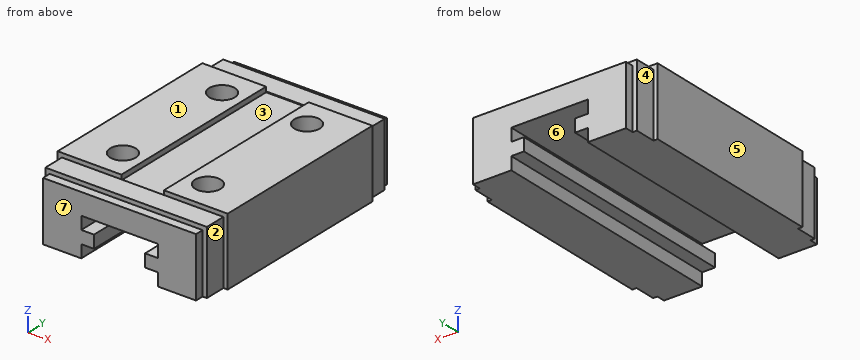
Autodesk Inventor part; units mm, degrees
ref_plane "YZ Plane" through (0, 0, 0) normal (1, 0, 0) x (0, 1, 0)
ref_plane "XZ Plane" through (0, 0, 0) normal (0, 1, 0) x (-1, 0, 0)
ref_plane "XY Plane" through (0, 0, 0) normal (0, 0, 1) x (1, 0, 0)
sketch "Szkic1" plane through (0, 0, 0) normal (0, 0, 1) x (1, 0, 0)
  line L0 (0, 0) -> (10, 0)
  line L1 (10, 0) -> (10, 28.9)
  line L2 (10, 28.9) -> (-10, 28.9)
  line L3 (-10, 28.9) -> (-10, 0)
  line L4 (-10, 0) -> (10, 0)
  dimension "d1" = 28.9
  dimension "d2" = 20
extrude "Wyciągnięcie proste1" add sketch "Szkic1" along normal blind 8
sketch "Szkic2" plane through (-10, 0, 0) normal (0, -1, 0) x (1, 0, 0)
  line L0 (0, 0) -> (20, 0)
  line L1 (20, 0) -> (20, 8)
  line L2 (0, 8) -> (20, 8)
  line L3 (0, 0) -> (0, 8)
  line L4 (14.5, 4.5) -> (5.5, 4.5)
  line L5 (14.5, 4.5) -> (14.5, 3)
  line L6 (14.5, 3) -> (13, 3)
  line L7 (13, 3) -> (13, 1.5)
  line L8 (13, 1.5) -> (14.5, 1.5)
  line L9 (5.5, 4.5) -> (5.5, 3)
  line L10 (5.5, 3) -> (7, 3)
  line L11 (7, 3) -> (7, 1.5)
  line L12 (7, 1.5) -> (5.5, 1.5)
  line L13 (5.5, 4.5) -> (5.5, 3)
  line L14 (5.5, 1.5) -> (5.5, 0)
  line L15 (14.5, 0) -> (14.5, 1.5)
  line L16 (14.5, 3) -> (14.5, 4.5)
extrude "Wyciągnięcie proste2" cut sketch "Szkic2" against normal up to next contours L14 L12 L11 L10 L9 L4 L5 L6 L7 L8 L15 L0
sketch "Szkic3" plane through (0, 0, 8) normal (0, 0, 1) x (1, 0, 0)
  line L0 (10, 0) -> (10, 28.9)
  line L1 (10, 28.9) -> (-10, 28.9)
  line L2 (-10, 28.9) -> (-10, 0)
  line L3 (-10, 0) -> (10, 0)
  line L4 (10, 28.9) -> (-10, 0)
  line L5 (10, 28.9) -> (-10, 28.9)
  line L6 (10, 0) -> (-10, 28.9)
  line L7 (-10, 28.9) -> (0, 14.45)
  line L8 (0, 14.45) -> (0, 6.95)
  line L9 (0, 6.95) -> (5, 6.95)
  line L10 (5, 6.95) -> (5, 21.95)
  line L11 (3, 0) -> (3, 28.9)
  line L12 (5, 21.95) -> (-5, 21.95)
  line L13 (-5, 21.95) -> (-5, 6.95)
  line L14 (-5, 6.95) -> (0, 6.95)
  line L15 (-3, 0) -> (-3, 28.9)
  circle A0 centre (5, 21.95) radius 1.5
  circle A1 centre (5, 6.95) radius 1.5
  circle A2 centre (-5, 21.95) radius 1.5
  circle A3 centre (-5, 6.95) radius 1.5
  point P0 (0, 0)
  dimension "d23" = 10
  dimension "d24" = 15
  dimension "d25" = 3
  dimension "d26" = 3
  dimension "d27" = 3
  dimension "d28" = 3
extrude "Wyciągnięcie proste3" cut sketch "Szkic3" against normal blind 3 contours A1 L9 L10 L6 | L6 L10 A1 | A0 L10 L4 | L4 L10 L12 A0 | L10 L9 A1 L6 | L6 A1 L10 | L10 A0 L4 | L4 A0 L12 L10 | A3 L13 L4 | L4 L13 L14 A3 | L14 L13 L4 A3 | A2 L12 L13 L6 | L6 L13 A2 | A2 L6 L13 L12 | L13 A3 L4 | L6 A2 L13
thread "Gwint1"
thread "Gwint2"
thread "Gwint3"
thread "Gwint4"
sketch "Szkic4" plane through (0, 0, 8) normal (0, 0, 1) x (1, 0, 0)
  circle A0 centre (-5, 6.95) radius 1.5
  circle A1 centre (5, 6.95) radius 1.5
  circle A2 centre (5, 21.95) radius 1.5
  circle A3 centre (-5, 21.95) radius 1.5
  line L0 (10, 28.9) -> (-10, 28.9)
  line L1 (-10, 0) -> (10, 0)
  line L2 (-10, 0) -> (-10, 1)
  line L3 (-10, 1) -> (10, 1)
  line L4 (-10, 28.9) -> (-10, 27.9)
  line L5 (-10, 27.9) -> (10, 27.9)
  line L6 (-10, 28.9) -> (-10, 27.9)
  line L7 (-10, 1) -> (-10, 0)
  line L8 (10, 0) -> (10, 1)
  line L9 (10, 27.9) -> (10, 28.9)
  line L10 (10, 0) -> (10, 1)
  line L11 (10, 27.9) -> (10, 28.9)
  line L12 (-10, 28.9) -> (-10, 27.9)
  line L13 (-10, 1) -> (-10, 0)
  point P0 (0, 0)
  dimension "d39" = 1
  dimension "d40" = 1
extrude "Wyciągnięcie proste4" cut sketch "Szkic4" against normal blind 1 contours L9 L5 L4 L0 | L2 L3 L8 L1
sketch "Szkic5" plane through (10, 0, 0) normal (1, 0, 0) x (0, 0, -1)
  line L0 (-7, 1) -> (-7, 0)
  line L1 (0, 0) -> (-7, 0)
  line L2 (0, 0) -> (0, 28.9)
  line L3 (-7, 28.9) -> (-7, 27.9)
  line L4 (0, 28.9) -> (-7, 28.9)
  line L5 (-7, 1) -> (0, 1)
  line L6 (-7, 27.9) -> (0, 27.9)
extrude "Wyciągnięcie proste5" cut sketch "Szkic5" against normal blind 1
sketch "Szkic6" plane through (-10, 0, 0) normal (-1, 0, 0) x (0, 0, 1)
  line L0 (7, 27.9) -> (7, 28.9)
  line L1 (0, 28.9) -> (7, 28.9)
  line L2 (0, 28.9) -> (0, 0)
  line L3 (0, 0) -> (7, 0)
  line L4 (7, 0) -> (7, 1)
  line L5 (8, 27.9) -> (7, 27.9)
  line L6 (7, 27.9) -> (0, 27.9)
  line L7 (7, 1) -> (0, 1)
extrude "Wyciągnięcie proste6" cut sketch "Szkic6" against normal blind 1
sketch "Szkic7" plane through (0, 0, 8) normal (0, 0, 1) x (1, 0, 0)
  circle A0 centre (-5, 21.95) radius 1.5
  circle A1 centre (5, 21.95) radius 1.5
  circle A2 centre (5, 6.95) radius 1.5
  circle A3 centre (-5, 6.95) radius 1.5
  line L0 (-10, 1) -> (10, 1)
  line L1 (10, 27.9) -> (-10, 27.9)
  line L2 (10, 27.9) -> (10, 25.4)
  line L3 (10, 25.4) -> (-10, 25.4)
  line L4 (10, 1) -> (9, 1)
  line L5 (10, 1) -> (10, 3.5)
  line L6 (10, 3.5) -> (-10, 3.5)
  line L7 (10, 1) -> (10, 3.5)
  line L8 (10, 25.4) -> (10, 27.9)
  line L9 (10, 1) -> (10, 3.5)
  line L10 (10, 25.4) -> (10, 27.9)
  line L11 (-10, 27.9) -> (-10, 25.4)
  line L12 (-10, 3.5) -> (-10, 1)
  line L13 (-10, 27.9) -> (-10, 25.4)
  line L14 (-10, 3.5) -> (-10, 1)
  point P0 (0, 0)
  dimension "d47" = 2.5
  dimension "d48" = 2.5
extrude "Wyciągnięcie proste7" cut sketch "Szkic7" against normal blind 0.5 contours L12 L6 L5 L0 | L2 L3 L11 L1
sketch "Szkic8" plane through (-10, 1, 0) normal (-1, 0, 0) x (0, 0, 1)
  line L0 (7.5, 24.4) -> (7.5, 26.9)
  line L1 (7.5, 26.9) -> (0, 26.9)
  line L2 (7.5, 0) -> (7.5, 2.5)
  line L3 (0, 0) -> (7.5, 0)
  line L4 (0, 26.9) -> (0, 0)
  line L5 (7.5, 24.4) -> (0, 24.4)
  line L6 (7.5, 2.5) -> (7.5, 0)
  line L7 (7.5, 2.5) -> (0, 2.5)
  point P0 (0, -1)
extrude "Wyciągnięcie proste8" cut sketch "Szkic8" against normal blind 0.5
sketch "Szkic9" plane through (10, 1, 0) normal (1, 0, 0) x (0, 0, -1)
  line L0 (-7.5, 2.5) -> (-7.5, 0)
  line L1 (-7.5, 0) -> (0, 0)
  line L2 (-7.5, 26.9) -> (-7.5, 24.4)
  line L3 (0, 26.9) -> (-7.5, 26.9)
  line L4 (0, 0) -> (0, 26.9)
  line L5 (0, 2.5) -> (-8, 2.5)
  line L6 (-7.5, 2.5) -> (0, 2.5)
  line L7 (-8, 24.4) -> (0, 24.4)
  line L8 (-7.5, 24.4) -> (0, 24.4)
  point P0 (0, -1)
extrude "Wyciągnięcie proste9" cut sketch "Szkic9" against normal blind 0.5
sketch "Szkic10" plane through (0, 0, 8) normal (0, 0, 1) x (1, 0, 0)
  line L0 (-10, 3.5) -> (10, 3.5)
  line L1 (10, 3.5) -> (10, 25.4)
  line L2 (10, 25.4) -> (-10, 25.4)
  line L3 (-10, 25.4) -> (-10, 3.5)
  circle A0 centre (-5, 21.95) radius 1.5
  circle A1 centre (5, 21.95) radius 1.5
  circle A2 centre (5, 6.95) radius 1.5
  circle A3 centre (-5, 6.95) radius 1.5
  line L4 (0, 3.5) -> (-2.5, 3.5)
  line L5 (-9.5, 3.5) -> (9.5, 3.5)
  line L6 (-2.5, 3.5) -> (-2.5, 25.4)
  line L7 (10, 25.4) -> (-10, 25.4)
  line L8 (-2.5, 25.4) -> (2.5, 25.4)
  line L9 (2.5, 25.4) -> (2.5, 3.5)
  line L10 (0, 3.5) -> (2.5, 3.5)
  point P0 (0, 0)
  dimension "d55" = 2.5
  dimension "d56" = 5
extrude "Wyciągnięcie proste10" cut sketch "Szkic10" against normal blind 0.6 contours L6 L2 L9 L0
properties part number "Wózel MGN9C"
Model file for the job. Use its own axes, mm. Face numbers are marked on the shaded views. A direction names the side the tool comes from. Give positions to 0.01 mm unless a question says otherwise; leave off trailing zeros. Write each loop counter-clockwise with the first axis right and the second up, starting at its lowest first coordinate (ties: lowest second). Pieces come first, ordered by that corner, then holes. Notation, with made-up numbers: (61, -15) -> (98, -15) arc R22 cw to (98, 10) -> close; hole circle Ø9 at (4, 3). An arc over 180 degrees is marked (long way). Write item = value, one per line.
(1) Tool access for the marked faces 1, 2, 3 and 4: list every direction of +Z, -Z, +X, -X, +Y, -Y with a clear straight run to the whole face (end or side of a thin tool).
Determined:
face_1 = +Z, +X, -X, +Y, -Y
face_2 = +Z, -Z, +X, -Y
face_3 = +Z
face_4 = +Z, -Z, -X, +Y
(2) Mould opens along X. For the marked faces 5, 6 and 7 say: released by +X, released by -X, zero draft, split by the parting line, or undercut.
Determined:
face_5 = released by -X
face_6 = undercut
face_7 = zero draft
(3) Slice it at A-A, the plane z = 2.5. Give the cut face in (x, y), then the cut area to 3 significant figures.
Determined:
outline = (-10, 3.5) -> (-9.5, 3.5) -> (-9.5, 1) -> (-9, 1) -> (-9, 0) -> (-3, 0) -> (-3, 28.9) -> (-9, 28.9) -> (-9, 27.9) -> (-9.5, 27.9) -> (-9.5, 25.4) -> (-10, 25.4) -> close; (3, 0) -> (9, 0) -> (9, 1) -> (9.5, 1) -> (9.5, 3.5) -> (10, 3.5) -> (10, 25.4) -> (9.5, 25.4) -> (9.5, 27.9) -> (9, 27.9) -> (9, 28.9) -> (3, 28.9) -> close
area = 396 mm2
(4) Slice it at D-D, the plane x = -1.75. Give the cut face in (y, z).
Determined:
outline = (0, 4.5) -> (28.9, 4.5) -> (28.9, 7) -> (27.9, 7) -> (27.9, 7.5) -> (25.4, 7.5) -> (25.4, 7.4) -> (3.5, 7.4) -> (3.5, 7.5) -> (1, 7.5) -> (1, 7) -> (0, 7) -> close
(5) Slice it at C-C, the plane y = 21.95. Give the cut face in (x, z), then the cut area to 3 significant figures.
Determined:
outline = (-10, 0) -> (-4.5, 0) -> (-4.5, 1.5) -> (-3, 1.5) -> (-3, 3) -> (-4.5, 3) -> (-4.5, 4.5) -> (4.5, 4.5) -> (4.5, 3) -> (3, 3) -> (3, 1.5) -> (4.5, 1.5) -> (4.5, 0) -> (10, 0) -> (10, 8) -> (6.5, 8) -> (6.5, 5) -> (3.5, 5) -> (3.5, 8) -> (2.5, 8) -> (2.5, 7.4) -> (-2.5, 7.4) -> (-2.5, 8) -> (-3.5, 8) -> (-3.5, 5) -> (-6.5, 5) -> (-6.5, 8) -> (-10, 8) -> close
area = 103 mm2
(6) Flat gauge pin, fed straight in: P1, Ø1.5, axis at x = -5, y = 6.5, coming from the +Z side. Where does the tip first touch, or does it go through?
Determined:
P1 = 5
(7) Probe line 1 along X through (y, z) = (21.95, 6.1); line 2 along X through (y, z) = (26.75, 2); line 3 along Z through (x, y) = (4, 26). List the from-to ranges inside material, lowest first.
Determined:
line_1 = -10 to -6.5, -3.5 to 3.5, 6.5 to 10
line_2 = -9.5 to -3, 3 to 9.5
line_3 = 1.5 to 3, 4.5 to 7.5
(8) Slice it at B-B, the plane z = 6. Give the cut face in (x, y).
Determined:
outline = (-10, 3.5) -> (-9.5, 3.5) -> (-9.5, 1) -> (-9, 1) -> (-9, 0) -> (9, 0) -> (9, 1) -> (9.5, 1) -> (9.5, 3.5) -> (10, 3.5) -> (10, 25.4) -> (9.5, 25.4) -> (9.5, 27.9) -> (9, 27.9) -> (9, 28.9) -> (-9, 28.9) -> (-9, 27.9) -> (-9.5, 27.9) -> (-9.5, 25.4) -> (-10, 25.4) -> close; hole circle Ø3 at (-5, 6.95); hole circle Ø3 at (-5, 21.95); hole circle Ø3 at (5, 6.95); hole circle Ø3 at (5, 21.95)
